Here's the drawing with two shaded views (mm, measured from the low corner). I have some questions. A direction names the side the tool comes from. Give positions to 0.01 mm unless a question says otherwise; leave off trailing zeros. Order: outer loops, then holes, each group sorted by start corner. A loop starts at its lowest first (then second) coordinate and runs counter-clockwise, first axis right, second up. Notation, with made-up numbers: M 19,21.25 L 36,21.25 A7 ccw 36,34.25 Z; hole C 62.25,70.25 d4. An arc over 180 degrees is marked long. One line per question, with ' | ' between items. Start each with the question number.
1) If we section it at B-B, the plane y = 43.5: Please give me the cut outline in (x, z).
2) I'm going to push a flat-ended pin straight in: pin 1 Ø6 at (x, y) = (61, 82) entering from +Z. Where does the tip first touch, or does it pass through?
3) If we section it at A-A, the plane z = 46: Please give me the cut outline in (x, y).
4) Thinking about a two-plate mould opening in X: for the marked faces 1, 2 and 3, which applies, +X half, -X half, draft (parallel to the pull), parting line (faces both ways), or undercut?
5) Please list where these lines run through material, in increasing order: line 1 along X through (y, z) = (62, 34); line 2 along Z through (x, y) = (22, 82). Write a range as [from, to].
6) For the marked faces 4, 5 and 6, which set-ups out of +Z, -Z, +X, -X, +Y, -Y let a thin tool reach every point of the face, with its end or its side?
7) If we section it at D-D, the plane x = 99.5: Please give me the cut outline in (y, z).
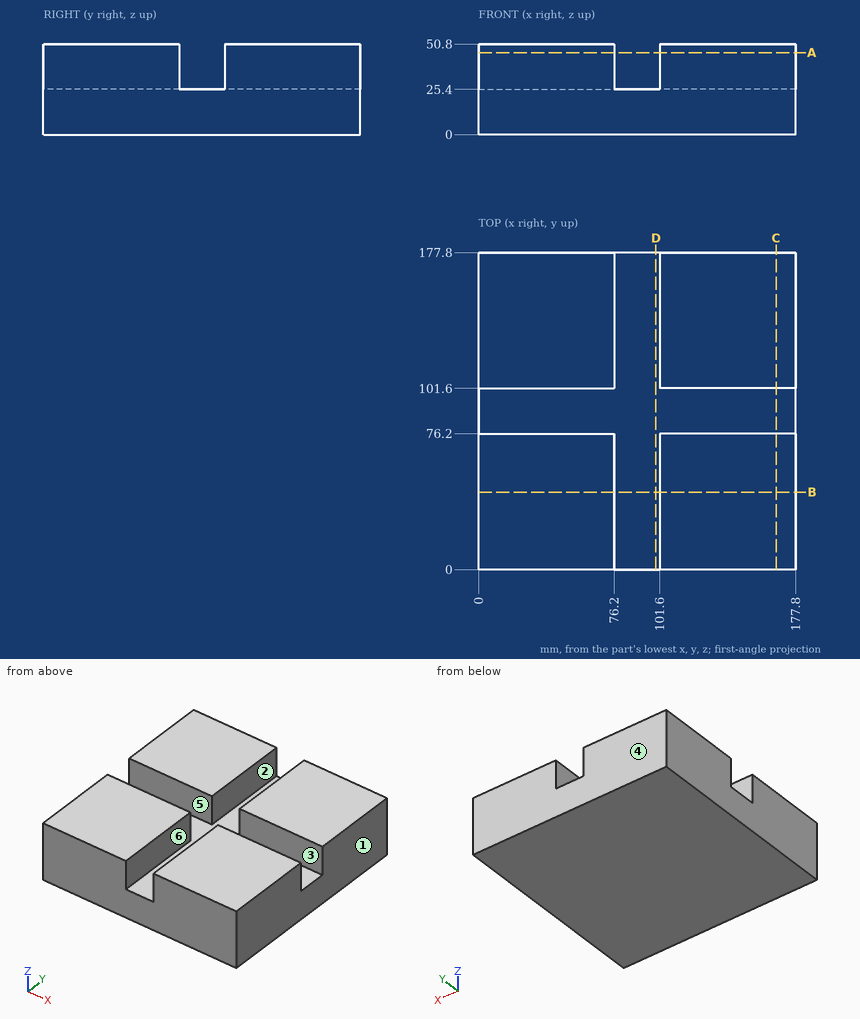
Results found:
1) outline: M 0,0 L 177.8,0 L 177.8,50.8 L 101.6,50.8 L 101.6,25.4 L 76.2,25.4 L 76.2,50.8 L 0,50.8 Z
2) pin 1: stops at z = 25.4
3) outline: M 0,0 L 76.2,0 L 76.2,76.2 L 0,76.2 Z; M 0,101.6 L 76.2,101.6 L 76.2,177.8 L 0,177.8 Z; M 101.6,0 L 177.8,0 L 177.8,76.2 L 101.6,76.2 Z; M 101.6,101.6 L 177.8,101.6 L 177.8,177.8 L 101.6,177.8 Z
4) face 1: +X half | face 2: undercut | face 3: draft
5) line 1: x = [0, 76.2], [101.6, 177.8] | line 2: z = [0, 25.4]
6) face 4: +Z, -Z, +X, -X, +Y | face 5: +Z, +X, -X | face 6: +Z, +Y, -Y
7) outline: M 0,0 L 177.8,0 L 177.8,25.4 L 0,25.4 Z
